from build123d import *

# Parameters (mm, degrees)
F0_R     = 8.5
F1_DEPTH = 4
F2_R     = 5
F3_DEPTH = 100


with BuildPart() as f1:
    # F0 (on Top) → F1 (new body)
    with BuildSketch(Plane.XY):
        Circle(F0_R)
    extrude(amount=F1_DEPTH)

    # F2 (on Top) → F3 (join)
    with BuildSketch(Plane.XY):
        Circle(F2_R)
    extrude(amount=F3_DEPTH)

    # F4 (on Right) → F5 (revolve)
    with BuildSketch(Plane.YZ):
        with BuildLine():
            Line((0, 100), (5, 100))
            ThreePointArc((5, 100), (3.535534, 103.535534), (0, 105))
            Line((0, 105), (0, 100))
        make_face()
    revolve(axis=Axis((0, 0, 102.5), (0, 0, -1)))


solid = f1.part
Model file for the job. Use its own axes, mm. A direction names the side the tool comes from. Round coordinates to 2 decimals unless told otherwise and drop trailing zeros. Loops run counter-clockwise (first coordinate to the right, second up) from the corner with the lowest first, then second, coordinate; pieces in that order, holes last.
1. Band-saw the part on B-B, the plane z = 45.5. List the corners of the cut face in (x, y), and give its area (3 significant figures).
Check values:
outline: circle Ø10 at (0, 0)
area: 78.5 mm2
2. Tool access for faces 1 (the cylindrical face through (-1.08, -4.88, 51.33)), 2 (the cylindrical face through (4.57, 7.167, 1.972)): list every direction of +Z, -Z, +X, -X, +Y, -Y with a clear straight run to the whole face (end or side of a thin tool).
Check values:
face 1: +Z
face 2: +Z, -Z
3. Band-saw the part on A-A, the plane x = 6.75. List the corners of the cut face in (y, z).
Check values:
outline: (-5.17, 0) - (5.17, 0) - (5.17, 4) - (-5.17, 4) - close
4. Drop flat-ended pins along their axis: P1, Ø1.5, axis at y = -4.5, z = 78.5, coming from the +X side; P2, Ø10, axis at x = 5.5, z = 81.5, coming from the -Y side; P3, Ø1.5, axis at x = 4.5, y = 2, coming from the +Z side. Give the stop position or say it passes through.
Check values:
P1: stops at x = 3.31
P2: stops at y = -4.97
P3: stops at z = 102.75
5. Wall check: probe 1 along X at (y, z) = (0.25, 83); probe 2 along Z at (x, y) = (7, -1); probe 3 along Y at (x, z) = (2, 65.5). Give the ranges that are in metal, low to high.
Check values:
probe 1: x = -4.99 to 4.99
probe 2: z = 0 to 4
probe 3: y = -4.58 to 4.58
